For this review, take the finished solid that the model builds, in its own axes (mm). Face numbers are marked on the shaded views. A direction names the side the tool comes from. Round coordinates to 2 decimals unless told otherwise and drop trailing zeros. Order: outer loops, then holes, each group sorted by start corner. A loop starts at its lowest first (then second) coordinate and runs counter-clockwise, first axis right, second up. Notation, with made-up numbers: M 53.5,-24 L 69.5,-24 A23 cw 69.5,6 Z; hole C 62.5,-2 d9. An arc over 180 degrees is marked long. Use a Markdown table: item, result.
from build123d import *

# Parameters (mm, degrees)
F0_W     = 24.0008160472
F0_H     = 14.9513203651
F0_W_2   = 16.1316711456
F0_H_2   = 2.3607341573
F0_W_3   = 56.2641583383
F2_DEPTH = 12.7
F4_DEPTH = 25.4


# Not quite as in the source:
# - the program builds the solid bodies; features that only make, move or delete a surface that nothing else refers to are left out


with BuildPart() as f2:
    # F0 (on Front) → F2 (new body, symmetric)
    with BuildSketch(Plane.XZ):
        with Locations((-3.7378184497, 0)):
            Rectangle(F0_W, F0_H)
        Polygon((24.3942607194, 34.2306494713), (-24.3942607194, 34.2306494713), (-24.3942607194, -34.2306494713), (24.3942607194, -34.2306494713), (24.3942607194, -9.8363943398), (8.2625895739, -9.8363943398), (8.2625895739, -7.4756601825), (-15.7382264733, -7.4756601825), (-15.7382264733, 7.4756601825), (8.2625895739, 7.4756601825), (8.2625895739, 9.8363943398), (24.3942607194, 9.8363943398), align=None)
        with Locations((32.4600962922, 0)):
            Rectangle(F0_W_2, F0_H)
        with Locations((16.3284251466, 0)):
            Rectangle(F0_W_2, F0_H)
        with Locations((16.3284251466, 8.6560272612)):
            Rectangle(F0_W_2, F0_H_2)
        with Locations((32.4600962922, 8.6560272612)):
            Rectangle(F0_W_2, F0_H_2)
        with Locations((16.3284251466, -8.6560272612)):
            Rectangle(F0_W_2, F0_H_2)
        with Locations((32.4600962922, -8.6560272612)):
            Rectangle(F0_W_2, F0_H_2)
        with Locations((68.6580110341, 0)):
            Rectangle(F0_W_3, F0_H)
    extrude(amount=F2_DEPTH, both=True)

    # F4 (add): a face of the model
    f4_faces = [f2.faces().sort_by_distance(p)[0] for p in [
        (15.1283797196, 12.7, 0),
    ]]
    extrude(f4_faces, amount=-F4_DEPTH)


solid = f2.part
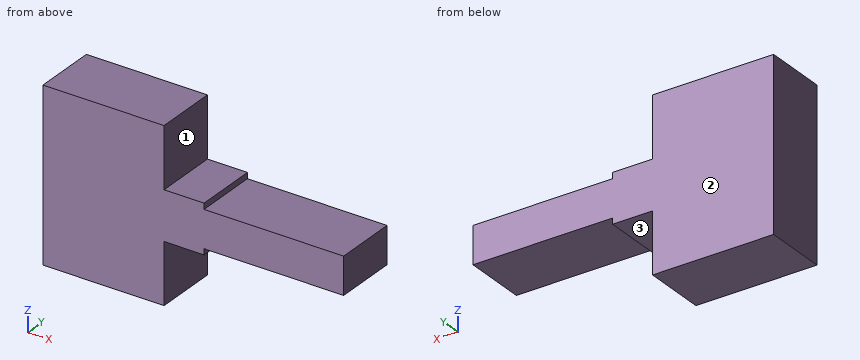
Q1. Add section A-A (y = 1). Write out the cut boundary in (x, z), then the cut area to 3 significant figures.
Determined:
| item | result |
|---|---|
| outline | M -24.39,-34.23 L 24.39,-34.23 L 24.39,-9.84 L 40.53,-9.84 L 40.53,-7.48 L 96.79,-7.48 L 96.79,7.48 L 40.53,7.48 L 40.53,9.84 L 24.39,9.84 L 24.39,34.23 L -24.39,34.23 Z |
| area | 4,500 mm^2 |
Q2. Add section B-B (z = 18). Write out the cut boundary in (x, y), then the cut area to 3 significant figures.
Determined:
| item | result |
|---|---|
| outline | M -24.39,-12.7 L 24.39,-12.7 L 24.39,12.7 L -24.39,12.7 Z |
| area | 1,240 mm^2 |
Q3. Wall thickness on line 1 along Z through (x, y) = (34.5, -10.25); line 2 along X through (y, z) = (2.5, -14.5); line 3 along Z through (x, y) = (51.5, 6.25): over which ranges is each line inside the solid? List them lowest first. Write a range as [from, to].
Determined:
| item | result |
|---|---|
| line 1 | z = [-9.84, 9.84] |
| line 2 | x = [-24.39, 24.39] |
| line 3 | z = [-7.48, 7.48] |
Q4. Clearance check with flat-ended pins moving along their axes: pin 1 (1.2 mm diameter, centred on y = -6, z = -8.5, fed in from +X); pin 2 (7.5 mm diameter, centred on x = 73.5, y = 2, fed in from -Z); pin 3 (8 mm diameter, centred on x = 31.5, y = 0, fed in from -Z). State where each tip first meets the part, or that it passes through.
Determined:
| item | result |
|---|---|
| pin 1 | stops at x = 40.53 |
| pin 2 | stops at z = -7.48 |
| pin 3 | stops at z = -9.84 |
Q5. Add section C-C (x = 56.5). Write out the cut boundary in (y, z).
Determined:
| item | result |
|---|---|
| outline | M -12.7,-7.48 L 12.7,-7.48 L 12.7,7.48 L -12.7,7.48 Z |
Q6. Machinability: for the marked faces 1, 2 and 3, which of the approach directions +Z, -Z, +X, -X, +Y, -Y give a long, thin tool a straight path to every point of the face, cutting with its end or side? Answer none if there is none.
Determined:
| item | result |
|---|---|
| face 1 | +Z, +X, +Y, -Y |
| face 2 | +Z, -Z, +X, -X, +Y |
| face 3 | -Z, +X, +Y, -Y |
